```python
from build123d import *

# Parameters (mm, degrees)
IZIM1_R                          = 18.5
Y_KSEKLIK_EKSTR_ZYON1_DEPTH      = 6.5
KES_EKSTR_ZYON1_DEPTH            = 6.5
Y_KSEKLIK_EKSTR_ZYON2_DEPTH      = 6.5
Y_KSEKLIK_EKSTR_ZYON3_DEPTH      = 30
Y_KSEKLIK_EKSTR_ZYON3_DEPTH_BACK = 6.5
IZIM4_W                          = 37
IZIM4_H                          = 4
IZIM5_W                          = 36.995441418
IZIM5_H                          = 250
Y_KSEKLIK_EKSTR_ZYON4_DEPTH      = 4
Y_KSEKLIK_EKSTR_ZYON6_DEPTH      = 6.5
Y_KSEKLIK_EKSTR_ZYON7_DEPTH      = 4
Y_KSEKLIK_EKSTR_ZYON8_DEPTH      = 6
IZIM15_W                         = 170.62151123
IZIM15_H                         = 260.400815818
KES_EKSTR_ZYON2_DEPTH            = 75.752098375
KES_EKSTR_ZYON3_DEPTH            = 8
IZIM17_W                         = 85.533609072
IZIM17_H                         = 320.477083545
KES_EKSTR_ZYON4_DEPTH            = 8
KES_EKSTR_ZYON5_DEPTH            = 8


with BuildPart() as part:
    # Çizim1 → Yükseklik-Ekstrüzyon1 (new body)
    with BuildSketch(Plane.XY):
        with Locations(Location((0, 0, 0), (0, 0, 180))):
            Circle(IZIM1_R)
    extrude(amount=Y_KSEKLIK_EKSTR_ZYON1_DEPTH)

    # Çizim2 → Kes-Ekstrüzyon1 (cut)
    with BuildSketch(Plane.XY.offset(6.5)):
        with BuildLine():
            Line((6.5, 0), (6.5, -7.5))
            ThreePointArc((6.5, -7.5), (0, -14), (-6.5, -7.5))
            Line((-6.5, -7.5), (-6.5, 0))
            Line((-6.5, 0), (6.5, 0))
        make_face()
        with BuildLine():
            Line((-16, 1.6), (-13.5, 1.6))
            ThreePointArc((-13.5, 1.6), (-11.9, 0), (-13.5, -1.6))
            Line((-13.5, -1.6), (-16, -1.6))
            ThreePointArc((-16, -1.6), (-17.6, 0), (-16, 1.6))
        make_face()
        with BuildLine():
            Line((16, -1.6), (13.5, -1.6))
            ThreePointArc((13.5, -1.6), (11.9, 0), (13.5, 1.6))
            Line((13.5, 1.6), (16, 1.6))
            ThreePointArc((16, 1.6), (17.6, 0), (16, -1.6))
        make_face()
        with BuildLine():
            Line((7.510154292, 16.186602557), (10.890511962, 13.897826987))
            ThreePointArc((10.890511962, 13.897826987), (11.31834042, 11.675899263), (9.096412696, 11.248070806))
            Line((9.096412696, 11.248070806), (5.716055026, 13.536846375))
            ThreePointArc((5.716055026, 13.536846375), (5.288226568, 15.758774099), (7.510154292, 16.186602557))
        make_face()
        with BuildLine():
            Line((-7.510154292, 16.186602557), (-10.890511962, 13.897826987))
            ThreePointArc((-10.890511962, 13.897826987), (-11.31834042, 11.675899263), (-9.096412696, 11.248070806))
            Line((-9.096412696, 11.248070806), (-5.716055026, 13.536846375))
            ThreePointArc((-5.716055026, 13.536846375), (-5.288226568, 15.758774099), (-7.510154292, 16.186602557))
        make_face()
    extrude(amount=-KES_EKSTR_ZYON1_DEPTH, mode=Mode.SUBTRACT)

    # Çizim3 → Yükseklik-Ekstrüzyon2 (add)
    with BuildSketch(Plane(origin=(0, 0, 0), x_dir=(-1, 0, 0), z_dir=(0, 0, -1))):
        with BuildLine():
            ThreePointArc((0, -18.5), (-13.081475452, -13.081475452), (-18.5, 0))
            Line((-18.5, 0), (-18.5, -18.5))
            Line((-18.5, -18.5), (0, -18.5))
        make_face()
        with BuildLine():
            Line((18.5, -18.5), (18.5, 0))
            ThreePointArc((18.5, 0), (13.081475452, -13.081475452), (0, -18.5))
            Line((0, -18.5), (18.5, -18.5))
        make_face()
    extrude(amount=-Y_KSEKLIK_EKSTR_ZYON2_DEPTH)

    # Çizim4 → Yükseklik-Ekstrüzyon3 (add, two sides: drawn at the far end of the back side and taken through both)
    with BuildSketch(Plane.XY.offset(6.5).offset(-Y_KSEKLIK_EKSTR_ZYON3_DEPTH_BACK)):
        with Locations((0, -20.5)):
            Rectangle(IZIM4_W, IZIM4_H)
    extrude(amount=Y_KSEKLIK_EKSTR_ZYON3_DEPTH + Y_KSEKLIK_EKSTR_ZYON3_DEPTH_BACK)

    # Çizim5 → Yükseklik-Ekstrüzyon4 (add)
    with BuildSketch(Plane.XZ.offset(22.5)):
        with Locations((-0.002279291, 125)):
            Rectangle(IZIM5_W, IZIM5_H)
    extrude(amount=-Y_KSEKLIK_EKSTR_ZYON4_DEPTH)

    # Çizim10 → Yükseklik-Ekstrüzyon6 (add)
    with BuildSketch(Plane.XY.offset(250)):
        with BuildLine():
            Line((-18.5, 0), (-18.5, -18.5))
            Line((-18.5, -18.5), (18.5, -18.5))
            Line((18.5, -18.5), (18.5, 0))
            ThreePointArc((18.5, 0), (0, 18.5), (-18.5, 0))
        make_face()
        with BuildLine():
            Line((5.716055026, 13.536846375), (9.096412696, 11.248070806))
            ThreePointArc((9.096412696, 11.248070806), (11.31834042, 11.675899263), (10.890511962, 13.897826987))
            Line((10.890511962, 13.897826987), (7.510154292, 16.186602557))
            ThreePointArc((7.510154292, 16.186602557), (5.288226568, 15.758774099), (5.716055026, 13.536846375))
        make_face(mode=Mode.SUBTRACT)
        with BuildLine():
            Line((-7.510154292, 16.186602557), (-10.890511962, 13.897826987))
            ThreePointArc((-10.890511962, 13.897826987), (-11.31834042, 11.675899263), (-9.096412696, 11.248070806))
            Line((-9.096412696, 11.248070806), (-5.716055026, 13.536846375))
            ThreePointArc((-5.716055026, 13.536846375), (-5.288226568, 15.758774099), (-7.510154292, 16.186602557))
        make_face(mode=Mode.SUBTRACT)
        with BuildLine():
            Line((-13.5, 1.6), (-16, 1.6))
            ThreePointArc((-16, 1.6), (-17.6, 0), (-16, -1.6))
            Line((-16, -1.6), (-13.5, -1.6))
            ThreePointArc((-13.5, -1.6), (-11.9, 0), (-13.5, 1.6))
        make_face(mode=Mode.SUBTRACT)
        with BuildLine():
            Line((6.5, -7.5), (6.5, 0))
            Line((6.5, 0), (-6.5, 0))
            Line((-6.5, 0), (-6.5, -7.5))
            ThreePointArc((-6.5, -7.5), (0, -14), (6.5, -7.5))
        make_face(mode=Mode.SUBTRACT)
        with BuildLine():
            Line((13.5, -1.6), (16, -1.6))
            ThreePointArc((16, -1.6), (17.6, 0), (16, 1.6))
            Line((16, 1.6), (13.5, 1.6))
            ThreePointArc((13.5, 1.6), (11.9, 0), (13.5, -1.6))
        make_face(mode=Mode.SUBTRACT)
    extrude(amount=-Y_KSEKLIK_EKSTR_ZYON6_DEPTH)

    # Çizim12 → Yükseklik-Ekstrüzyon7 (add)
    with BuildSketch(Plane(origin=(0, -18.5, 0), x_dir=(1, 0, 0), z_dir=(0, 1, 0))):
        with BuildLine():
            Line((-18.5, 0), (-18.5, -250))
            ThreePointArc((-18.5, -250), (-136.505823788, -125), (-18.5, 0))
        make_face()
    extrude(amount=-Y_KSEKLIK_EKSTR_ZYON7_DEPTH)

    # Çizim14 → Yükseklik-Ekstrüzyon8 (add)
    with BuildSketch(Plane.XZ.offset(22.5)):
        with BuildLine():
            Line((18.5, 36.5), (18.495441418, 36.5))
            Line((18.495441418, 36.5), (18.495441418, 250))
            Line((18.495441418, 250), (-18.5, 250))
            ThreePointArc((-18.5, 250), (-136.505823788, 125), (-18.5, 0))
            Line((-18.5, 0), (18.5, 0))
            Line((18.5, 0), (18.5, 36.5))
        make_face()
    extrude(amount=Y_KSEKLIK_EKSTR_ZYON8_DEPTH)

    # Çizim15 → Kes-Ekstrüzyon2 (cut)
    with BuildSketch(Plane(origin=(0, -18.5, 0), x_dir=(1, 0, 0), z_dir=(0, 1, 0))):
        with Locations((-103.810755615, -130.200407909)):
            Rectangle(IZIM15_W, IZIM15_H)
    extrude(amount=-KES_EKSTR_ZYON2_DEPTH, mode=Mode.SUBTRACT)

    # Çizim16 → Kes-Ekstrüzyon3 (cut)
    with BuildSketch(Plane.XZ.offset(28.5)):
        Polygon((-18.5, 250), (-18.5, 0), (18.5, 0), (18.5, 36.5), (18.495441418, 36.5), (18.495441418, 250), align=None)
    extrude(amount=-KES_EKSTR_ZYON3_DEPTH, mode=Mode.SUBTRACT)

    # Çizim17 → Kes-Ekstrüzyon4 (cut)
    with BuildSketch(Plane(origin=(0, -18.5, 0), x_dir=(1, 0, 0), z_dir=(0, 1, 0))):
        with Locations((24.266804536, -83.261458228)):
            Rectangle(IZIM17_W, IZIM17_H)
    extrude(amount=-KES_EKSTR_ZYON4_DEPTH, mode=Mode.SUBTRACT)


with BuildPart() as kes_ekstr_zyon4_piece_1:
    # of the separate pieces the step leaves, piece 1, a body of its own (kes_ekstr_zyon4_pieces)
    add(part.part.solids().sort_by_distance((-18.5, 0, 243.5))[0])

    # Çizim18 → Kes-Ekstrüzyon5 (cut)
    with BuildSketch(Plane(origin=(0, 0, 243.5), x_dir=(-1, 0, 0), z_dir=(0, 0, -1))):
        with BuildLine():
            Line((-18.5, 0), (-18.5, -18.5))
            Line((-18.5, -18.5), (-18.495441418, -18.5))
            Line((-18.495441418, -18.5), (-18.495441418, -20.5))
            Line((-18.495441418, -20.5), (18.5, -20.5))
            Line((18.5, -20.5), (18.5, 0))
            ThreePointArc((18.5, 0), (0, 18.5), (-18.5, 0))
        make_face()
    extrude(amount=-KES_EKSTR_ZYON5_DEPTH, mode=Mode.SUBTRACT)


with BuildPart() as kes_ekstr_zyon4_piece_2:
    # of the separate pieces the step leaves, piece 2, a body of its own (kes_ekstr_zyon4_pieces)
    add(part.part.solids().sort_by_distance((-18.5, 0, 0))[0])


solid = kes_ekstr_zyon4_piece_2.part
```
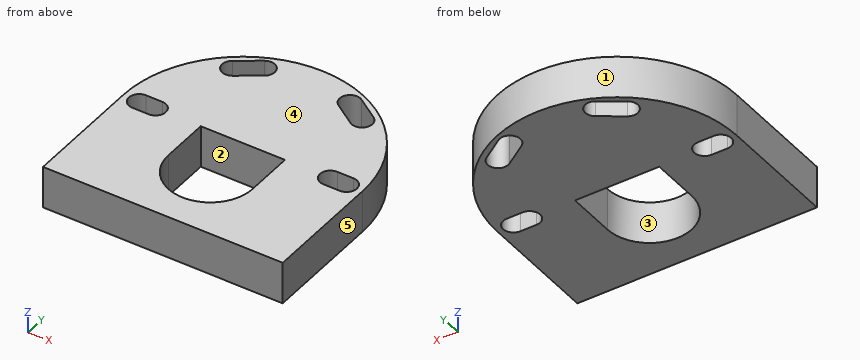
Source: CAD feature listing. Evaluate the final solid. Frame: model axes, mm. Face numbers are marked on the shaded views. A direction names the side the tool comes from. Coordinates: 2 decimals unless noted, no trailing zeros. Loops run counter-clockwise (first coordinate to the right, second up) from the corner with the lowest first, then second, coordinate; pieces in that order, holes last. Notation, with made-up numbers: (65, -22.5) - (123, -22.5) arc R16 ccw to (123, 7.5) - close; hole circle Ø10 at (24.25, -1.75). An arc over 180 degrees is marked (long way). Answer as CSV lines item,"result".
1. Section A-A (x = 0). Return loops of the section in (y, z).
Established:
outline,"(-18.5, 0) - (-14, 0) - (-14, 6.5) - (-18.5, 6.5) - close; (0, 0) - (18.5, 0) - (18.5, 6.5) - (0, 6.5) - close"
2. Section B-B (z = 0.5). Return loops of the section in (x, y).
Established:
outline,"(-18.5, -18.5) - (18.5, -18.5) - (18.5, 0) arc R18.5 ccw to (-18.5, 0) - close; hole (-16, -1.6) - (-13.5, -1.6) arc R1.6 ccw to (-13.5, 1.6) - (-16, 1.6) arc R1.6 ccw to start; hole (-10.89, 13.9) arc R1.6 ccw to (-9.1, 11.25) - (-5.72, 13.54) arc R1.6 ccw to (-7.51, 16.19) - close; hole (-6.5, -7.5) arc R6.5 ccw to (6.5, -7.5) - (6.5, 0) - (-6.5, 0) - close; hole (5.72, 13.54) - (9.1, 11.25) arc R1.6 ccw to (10.89, 13.9) - (7.51, 16.19) arc R1.6 ccw to start; hole (13.5, -1.6) - (16, -1.6) arc R1.6 ccw to (16, 1.6) - (13.5, 1.6) arc R1.6 ccw to start"
3. Section C-C (y = -10.5). Return loops of the section in (x, z), then the cut area to 3 significant figures.
Established:
outline,"(-18.5, 0) - (-5.77, 0) - (-5.77, 6.5) - (-18.5, 6.5) - close; (5.77, 0) - (18.5, 0) - (18.5, 6.5) - (5.77, 6.5) - close"
area,"166 mm2"
4. Contact query for flat-ended pins moving along their axis: pin 1 (3 mm diameter, centred on x = -15, z = 3, fed in from +Y); pin 2 (1.2 mm diameter, centred on x = 15, z = 2, fed in from +Y). Output: stop coordinate, or through.
Established:
pin 1,"stops at y = 12.65"
pin 2,"stops at y = 11.61"
5. Mould query, pull axis X, two halves, no side actions, for the marked faces 3, 4 and 5. Classes: released by +X, released by -X, zero draft, split by the parting line, or undercut.
Established:
face 3,"undercut"
face 4,"zero draft"
face 5,"released by +X"
6. Ray query, line 1 (X direction, y = -4, z = 3.25); line 2 (Y direction, x = 6, z = 4); line 3 (X direction, y = 14, z = 3). Return the intervals inside material, ascending.
Established:
line 1,"x = -18.5 to -6.5, 6.5 to 18.5"
line 2,"y = -18.5 to -10, 0 to 13.34, 16.34 to 17.5"
line 3,"x = -12.09 to -10.74, -5.26 to 5.26, 10.74 to 12.09"
7. Reachability of the marked faces 1 and 2 from +Z, -Z, +X, -X, +Y, -Y: full face, straight path, thin tool, end or side. Return the list, or none.
Established:
face 1,"+Z, -Z, +Y"
face 2,"+Z, -Z"
